Design review of the part built by this model. Coordinates are the model's own, in mm. Face numbers are marked on the shaded views. A direction names the side the tool comes from. Coordinates: 2 decimals unless noted, no trailing zeros. Order: outer loops, then holes, each group sorted by start corner. A loop starts at its lowest first (then second) coordinate and runs counter-clockwise, first axis right, second up.
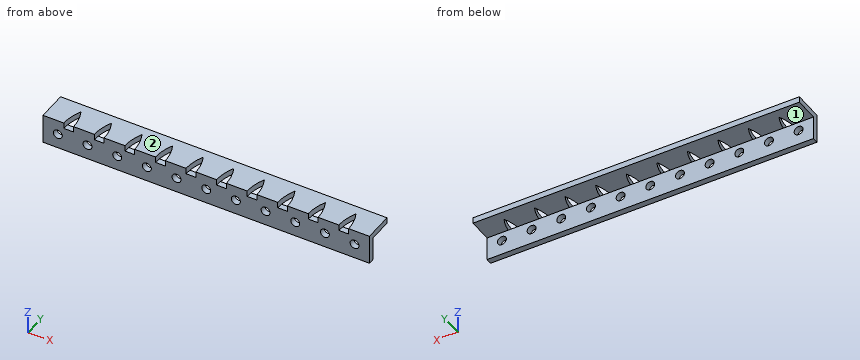
from build123d import *

# Parameters (mm, degrees)
SKETCH1_W                      = 110
SKETCH1_H                      = 10
SKETCH1_R                      = 1.5025
BOSS_EXTRUDE1_DEPTH            = 10
CUT_EXTRUDE1_REACH             = 7
SKETCH2_W                      = 110
SKETCH2_H                      = 8
CUT_EXTRUDE1_DIRECTION_2_DEPTH = 3
CUT_EXTRUDE2_DEPTH             = 2


with BuildPart() as part:
    # Sketch1 → Boss-Extrude1 (new body)
    with BuildSketch(Plane(origin=(0, 0, 0), x_dir=(1, 0, 0), z_dir=(0, 1, 0))):
        Rectangle(SKETCH1_W, SKETCH1_H)
        with Locations((-50, 0)):
            Circle(SKETCH1_R, mode=Mode.SUBTRACT)
        with Locations((-40, 0)):
            Circle(SKETCH1_R, mode=Mode.SUBTRACT)
        with Locations((-30, 0)):
            Circle(SKETCH1_R, mode=Mode.SUBTRACT)
        with Locations((-20, 0)):
            Circle(SKETCH1_R, mode=Mode.SUBTRACT)
        with Locations((-10, 0)):
            Circle(SKETCH1_R, mode=Mode.SUBTRACT)
        Circle(SKETCH1_R, mode=Mode.SUBTRACT)
        with Locations((10, 0)):
            Circle(SKETCH1_R, mode=Mode.SUBTRACT)
        with Locations((20, 0)):
            Circle(SKETCH1_R, mode=Mode.SUBTRACT)
        with Locations((30, 0)):
            Circle(SKETCH1_R, mode=Mode.SUBTRACT)
        with Locations((40, 0)):
            Circle(SKETCH1_R, mode=Mode.SUBTRACT)
        with Locations((50, 0)):
            Circle(SKETCH1_R, mode=Mode.SUBTRACT)
    extrude(amount=BOSS_EXTRUDE1_DEPTH)

    # Sketch2 → Cut-Extrude1 (cut, up to next)
    with BuildSketch(Plane.XY, mode=Mode.PRIVATE) as cut_extrude1_sk1:
        with Locations((0, 6)):
            Rectangle(SKETCH2_W, SKETCH2_H)
    cut_extrude1_tool1 = extrude(cut_extrude1_sk1.sketch, amount=-CUT_EXTRUDE1_REACH, mode=Mode.PRIVATE) & part.part
    add(cut_extrude1_tool1.solids().sort_by_distance((0, 6, 0))[0], mode=Mode.SUBTRACT)

    # Sketch2 → Cut-Extrude1 direction 2 (cut)
    with BuildSketch(Plane.XY):
        with Locations((0, 6)):
            Rectangle(SKETCH2_W, SKETCH2_H)
    extrude(amount=CUT_EXTRUDE1_DIRECTION_2_DEPTH, mode=Mode.SUBTRACT)

    # Sketch3 → Cut-Extrude2 (cut)
    with BuildSketch(Plane.XY.offset(5)):
        with BuildLine():
            Line((-37.7, 0), (-34.4, 0))
            add(Edge.make_bspline(
                [(-36.05, 7), (-34.434888234, 3.724961413), (-34.4, 0)],
                knots=[0, 0, 0, 1, 1, 1], degree=2))
            add(Edge.make_bspline(
                [(-36.05, 7), (-37.665111766, 3.724961413), (-37.7, 0)],
                knots=[0, 0, 0, 1, 1, 1], degree=2))
        make_face()
        with BuildLine():
            Line((-48, 0), (-44.7, 0))
            add(Edge.make_bspline(
                [(-46.35, 7), (-44.734888234, 3.724961413), (-44.7, 0)],
                knots=[0, 0, 0, 1, 1, 1], degree=2))
            add(Edge.make_bspline(
                [(-46.35, 7), (-47.965111766, 3.724961413), (-48, 0)],
                knots=[0, 0, 0, 1, 1, 1], degree=2))
        make_face()
        with BuildLine():
            Line((-27.4, 0), (-24.1, 0))
            add(Edge.make_bspline(
                [(-25.75, 7), (-24.134888234, 3.724961413), (-24.1, 0)],
                knots=[0, 0, 0, 1, 1, 1], degree=2))
            add(Edge.make_bspline(
                [(-25.75, 7), (-27.365111766, 3.724961413), (-27.4, 0)],
                knots=[0, 0, 0, 1, 1, 1], degree=2))
        make_face()
        with BuildLine():
            Line((-17.1, 0), (-13.8, 0))
            add(Edge.make_bspline(
                [(-15.45, 7), (-13.834888234, 3.724961413), (-13.8, 0)],
                knots=[0, 0, 0, 1, 1, 1], degree=2))
            add(Edge.make_bspline(
                [(-15.45, 7), (-17.065111766, 3.724961413), (-17.1, 0)],
                knots=[0, 0, 0, 1, 1, 1], degree=2))
        make_face()
        with BuildLine():
            Line((-6.8, 0), (-3.5, 0))
            add(Edge.make_bspline(
                [(-5.15, 7), (-3.534888234, 3.724961413), (-3.5, 0)],
                knots=[0, 0, 0, 1, 1, 1], degree=2))
            add(Edge.make_bspline(
                [(-5.15, 7), (-6.765111766, 3.724961413), (-6.8, 0)],
                knots=[0, 0, 0, 1, 1, 1], degree=2))
        make_face()
        with BuildLine():
            Line((3.5, 0), (6.8, 0))
            add(Edge.make_bspline(
                [(5.15, 7), (6.765111766, 3.724961413), (6.8, 0)],
                knots=[0, 0, 0, 1, 1, 1], degree=2))
            add(Edge.make_bspline(
                [(5.15, 7), (3.534888234, 3.724961413), (3.5, 0)],
                knots=[0, 0, 0, 1, 1, 1], degree=2))
        make_face()
        with BuildLine():
            Line((13.8, 0), (17.1, 0))
            add(Edge.make_bspline(
                [(15.45, 7), (17.065111766, 3.724961413), (17.1, 0)],
                knots=[0, 0, 0, 1, 1, 1], degree=2))
            add(Edge.make_bspline(
                [(15.45, 7), (13.834888234, 3.724961413), (13.8, 0)],
                knots=[0, 0, 0, 1, 1, 1], degree=2))
        make_face()
        with BuildLine():
            Line((24.1, 0), (27.4, 0))
            add(Edge.make_bspline(
                [(25.75, 7), (27.365111766, 3.724961413), (27.4, 0)],
                knots=[0, 0, 0, 1, 1, 1], degree=2))
            add(Edge.make_bspline(
                [(25.75, 7), (24.134888234, 3.724961413), (24.1, 0)],
                knots=[0, 0, 0, 1, 1, 1], degree=2))
        make_face()
        with BuildLine():
            Line((34.4, 0), (37.7, 0))
            add(Edge.make_bspline(
                [(36.05, 7), (37.665111766, 3.724961413), (37.7, 0)],
                knots=[0, 0, 0, 1, 1, 1], degree=2))
            add(Edge.make_bspline(
                [(36.05, 7), (34.434888234, 3.724961413), (34.4, 0)],
                knots=[0, 0, 0, 1, 1, 1], degree=2))
        make_face()
        with BuildLine():
            Line((44.7, 0), (48, 0))
            add(Edge.make_bspline(
                [(46.35, 7), (47.965111766, 3.724961413), (48, 0)],
                knots=[0, 0, 0, 1, 1, 1], degree=2))
            add(Edge.make_bspline(
                [(46.35, 7), (44.734888234, 3.724961413), (44.7, 0)],
                knots=[0, 0, 0, 1, 1, 1], degree=2))
        make_face()
    extrude(amount=-CUT_EXTRUDE2_DEPTH, mode=Mode.SUBTRACT)


solid = part.part
1. Add section A-A (x = -10). Give the boundary of the cut face in (y, z), and give its area (3 significant figures).
2. For the marked faces 1 and 2, list the 3-axis set-ups (+Z, -Z, +X, -X, +Y, -Y) from which the entire face can be reached by the end or side of a thin tool; tool diameter is ignored.
3. Add section C-C (z = -3.5). Give the boundary of the cut face in (x, y).
4. Add section B-B (y = 4.5). State how many separate pieces and enclosed holes the cut face has, and give its area (3 significant figures).
5. To check wall thickness, follow line 1 (Z direction, x = 40, y = 0.7); line 2 (Y direction, x = 31, z = -4.5); line 3 (Z direction, x = 28, y = 2.25). State the ranges of each line that lie inside material, in increasing order.
6. Insertion check: pin 1 (2 mm diameter, centred on x = -36.5, y = 0.5, fed in from +Z); pin 2 (2.5 mm diameter, centred on x = -18, y = 5, fed in from -Z). Each pin has a flat end and moves straight along its axis. Give the tip position at first contact, or say it passes through.
Solution:
1. outline: (0, -5) - (2, -5) - (2, -1.5) - (0, -1.5) - close; (0, 1.5) - (2, 1.5) - (2, 3) - (10, 3) - (10, 5) - (0, 5) - close
1. area: 30.0 mm2
2. face 1: -Z, +X, -X, +Y
2. face 2: +Z, +X, -X, +Y, -Y
3. outline: (-55, 0) - (55, 0) - (55, 2) - (-55, 2) - close
4. separate pieces: 11
4. enclosed holes: 0
4. area: 181 mm2
5. line 1: z = -5 to -1.5, 1.5 to 5
5. line 2: y = 0 to 2
5. line 3: z = 3 to 5
6. pin 1: stops at z = 3
6. pin 2: stops at z = 3
